Work out the finished part from the listing and answer in its coordinate system (mm). Give positions to 0.01 mm unless a question says otherwise; leave off trailing zeros. Loops run counter-clockwise (first coordinate to the right, second up) from the corner with the lowest first, then second, coordinate; pieces in that order, holes last.
```python
from build123d import *

# Parameters (mm, degrees)
F0_R     = 5
F1_DEPTH = 8.4
F2_SIZE  = 0.75
F3_F1_R  = 0.75
F3_F2_R  = 0.75
F3_F3_R  = 0.75
F3_F4_R  = 0.75
F3_F5_R  = 0.75
F3_F6_R  = 0.75
F3_F7_R  = 0.75
F3_F8_R  = 0.75
F3_F9_R  = 0.75
F3_F10_R = 0.75
F3_F11_R = 0.75
F3_F12_R = 0.75
F3_F13_R = 0.75
F3_F14_R = 0.75
F3_F15_R = 0.75
F3_F16_R = 0.75
F3_F17_R = 0.75
F3_F18_R = 0.75


with BuildPart() as f1:
    # F0 (on Top) → F1 (new body)
    with BuildSketch(Plane.XY):
        Polygon((4.6188021535, 8), (-4.6188021535, 8), (-9.237604307, 0), (-4.6188021535, -8), (4.6188021535, -8), (9.237604307, 0), align=None)
        Circle(F0_R, mode=Mode.SUBTRACT)
    extrude(amount=F1_DEPTH)

    # F2
    f2_edges = [f1.edges().sort_by_distance(p)[0] for p in [
        (0, -8, 8.4),
        (-6.928203, -4, 8.4),
        (-6.928203, 4, 8.4),
        (0, 8, 8.4),
        (6.928203, 4, 8.4),
        (6.928203, -4, 8.4),
        (6.928203, -4, 0),
        (0, -8, 0),
        (-6.928203, -4, 0),
        (-6.928203, 4, 0),
        (0, 8, 0),
        (6.928203, 4, 0),
    ]]
    chamfer(f2_edges, length=F2_SIZE)

    # F3: fillet of radius 0.75 on 18 edges, made by hand

    # F3_f1
    f3_f1_edges = [f1.edges().sort_by_distance(p)[0] for p in [
        (4.6188021535, 8, 4.2),
    ]]
    fillet(f3_f1_edges, radius=F3_F1_R)

    # F3_f2
    f3_f2_edges = [f1.edges().sort_by_distance(p)[0] for p in [
        (-4.6188021535, 8, 4.2),
    ]]
    fillet(f3_f2_edges, radius=F3_F2_R)

    # F3_f3
    f3_f3_edges = [f1.edges().sort_by_distance(p)[0] for p in [
        (9.237604307, 0, 4.2),
    ]]
    fillet(f3_f3_edges, radius=F3_F3_R)

    # F3_f4
    f3_f4_edges = [f1.edges().sort_by_distance(p)[0] for p in [
        (4.3732894516, 7.5747595264, 0.3247595264),
    ]]
    fillet(f3_f4_edges, radius=F3_F4_R)

    # F3_f5
    f3_f5_edges = [f1.edges().sort_by_distance(p)[0] for p in [
        (-4.3732894516, 7.5747595264, 0.3247595264),
    ]]
    fillet(f3_f5_edges, radius=F3_F5_R)

    # F3_f6
    f3_f6_edges = [f1.edges().sort_by_distance(p)[0] for p in [
        (4.3732894516, 7.5747595264, 8.0752404736),
    ]]
    fillet(f3_f6_edges, radius=F3_F6_R)

    # F3_f7
    f3_f7_edges = [f1.edges().sort_by_distance(p)[0] for p in [
        (-4.3732894516, 7.5747595264, 8.0752404736),
    ]]
    fillet(f3_f7_edges, radius=F3_F7_R)

    # F3_f8
    f3_f8_edges = [f1.edges().sort_by_distance(p)[0] for p in [
        (-9.237604307, 0, 4.2),
    ]]
    fillet(f3_f8_edges, radius=F3_F8_R)

    # F3_f9
    f3_f9_edges = [f1.edges().sort_by_distance(p)[0] for p in [
        (4.6188021535, -8, 4.2),
    ]]
    fillet(f3_f9_edges, radius=F3_F9_R)

    # F3_f10
    f3_f10_edges = [f1.edges().sort_by_distance(p)[0] for p in [
        (8.7465789032, 0, 0.3247595264),
    ]]
    fillet(f3_f10_edges, radius=F3_F10_R)

    # F3_f11
    f3_f11_edges = [f1.edges().sort_by_distance(p)[0] for p in [
        (8.7465789032, 0, 8.0752404736),
    ]]
    fillet(f3_f11_edges, radius=F3_F11_R)

    # F3_f12
    f3_f12_edges = [f1.edges().sort_by_distance(p)[0] for p in [
        (-8.7465789032, 0, 0.3247595264),
    ]]
    fillet(f3_f12_edges, radius=F3_F12_R)

    # F3_f13
    f3_f13_edges = [f1.edges().sort_by_distance(p)[0] for p in [
        (-8.7465789032, 0, 8.0752404736),
    ]]
    fillet(f3_f13_edges, radius=F3_F13_R)

    # F3_f14
    f3_f14_edges = [f1.edges().sort_by_distance(p)[0] for p in [
        (-4.6188021535, -8, 4.2),
    ]]
    fillet(f3_f14_edges, radius=F3_F14_R)

    # F3_f15
    f3_f15_edges = [f1.edges().sort_by_distance(p)[0] for p in [
        (4.3732894516, -7.5747595264, 0.3247595264),
    ]]
    fillet(f3_f15_edges, radius=F3_F15_R)

    # F3_f16
    f3_f16_edges = [f1.edges().sort_by_distance(p)[0] for p in [
        (4.3732894516, -7.5747595264, 8.0752404736),
    ]]
    fillet(f3_f16_edges, radius=F3_F16_R)

    # F3_f17
    f3_f17_edges = [f1.edges().sort_by_distance(p)[0] for p in [
        (-4.3732894516, -7.5747595264, 0.3247595264),
    ]]
    fillet(f3_f17_edges, radius=F3_F17_R)

    # F3_f18
    f3_f18_edges = [f1.edges().sort_by_distance(p)[0] for p in [
        (-4.3732894516, -7.5747595264, 8.0752404736),
    ]]
    fillet(f3_f18_edges, radius=F3_F18_R)


solid = f1.part
```
Q1. Consider line 1 along Y through (x, z) = (0, 6); line 2 along X through (y, z) = (4, 4.5); line 3 along X through (y, z) = (-1.5, 7.75). Determine where each line is inside the solid, lowest interval first.
Q2. Section A-A on y = 0 is taken. Give the vertices of the cut face in (x, z), plus the area to 3 significant figures.
Q3. Section C-C on z = 4.25 is taken. Give the vertices of the cut face in (x, y) (3 decimals).
Q4. Section D-D on y = 5.5 is taken. Give the vertices of the cut face in (x, z).
Q5. Section B-B on x = 0 is taken. Give the vertices of the cut face in (y, z), plus the area to 3 significant figures.
Q6. Given pin 1 (4 mm diameter, centred on x = -7.5, z = 3, fed in from +Y); pin 2 (6 mm diameter, centred on x = 0, y = 0, fed in from -Z); pin 3 (1 mm diameter, centred on x = -6.5, z = 4.5, fed in from -Y), each flat-ended and moving along its own axis, determine where each tip first touches the part or whether it passes through.
Check result:
1. line 1: y = -8 to -5, 5 to 8
1. line 2: x = -6.93 to -3, 3 to 6.93
1. line 3: x = -8.26 to -4.77, 4.77 to 8.26
2. outline: (-9.12, 0.72) - (-8.29, 0) - (-5, 0) - (-5, 8.4) - (-8.29, 8.4) - (-9.12, 7.68) - close; (5, 0) - (8.29, 0) - (9.12, 0.72) - (9.12, 7.68) - (8.29, 8.4) - (5, 8.4) - close
2. area: 68.1 mm2
3. outline: (-9.021, -0.375) - (-4.835, -7.625) arc R0.75 ccw to (-4.186, -8) - (4.186, -8) arc R0.75 ccw to (4.835, -7.625) - (9.021, -0.375) arc R0.75 ccw to (9.021, 0.375) - (4.835, 7.625) arc R0.75 ccw to (4.186, 8) - (-4.186, 8) arc R0.75 ccw to (-4.835, 7.625) - (-9.021, 0.375) arc R0.75 ccw to start; hole circle Ø10 at (0, 0)
4. outline: (-6.06, 0.75) - (-5.2, 0) - (5.2, 0) - (6.06, 0.75) - (6.06, 7.65) - (5.2, 8.4) - (-5.2, 8.4) - (-6.06, 7.65) - close
5. outline: (-8, 0.75) - (-7.25, 0) - (-5, 0) - (-5, 8.4) - (-7.25, 8.4) - (-8, 7.65) - close; (5, 0) - (7.25, 0) - (8, 0.75) - (8, 7.65) - (7.25, 8.4) - (5, 8.4) - close
5. area: 49.3 mm2
6. pin 1: stops at y = 6.47
6. pin 2: passes through
6. pin 3: stops at y = -5.61
